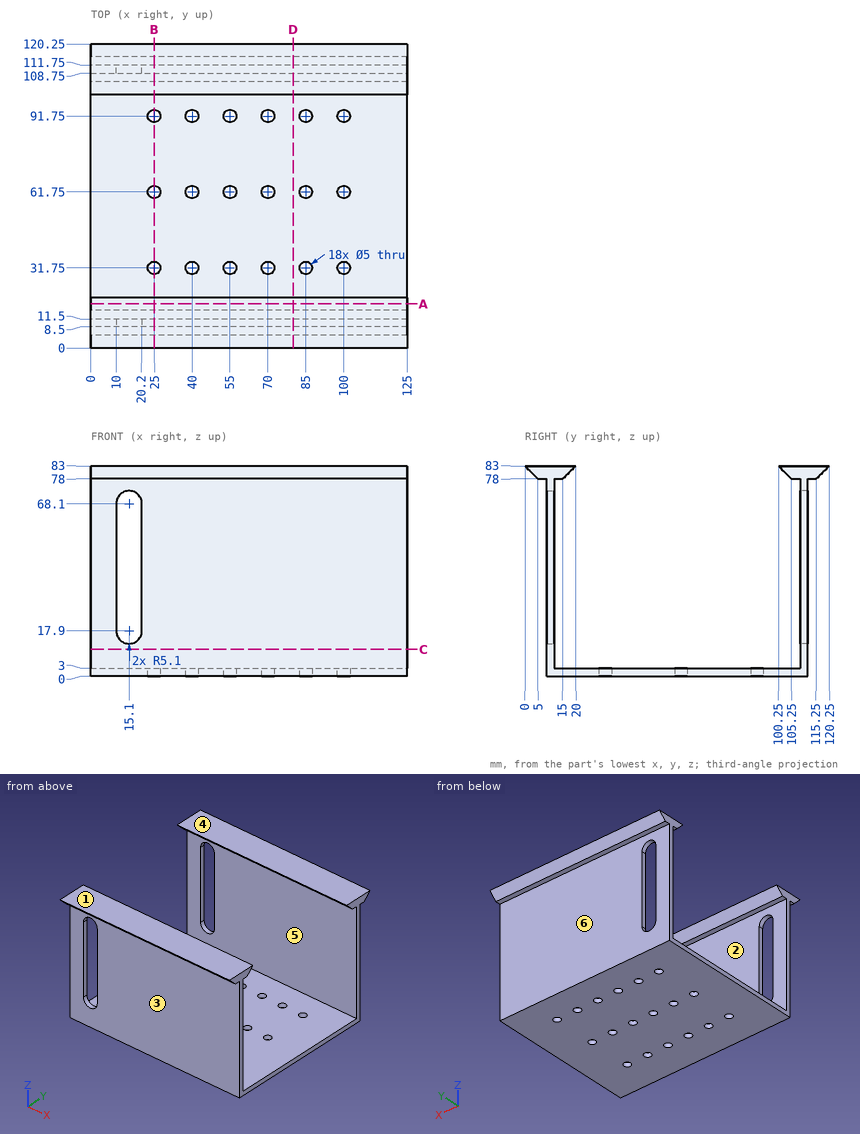
Source: three-view drawing plus pictorial views. Frame: mm from the lowest corner of the part. A direction names the side the tool comes from. Give positions to 0.01 mm unless a question says otherwise; leave off trailing zeros. Loops run counter-clockwise (first coordinate to the right, second up) from the corner with the lowest first, then second, coordinate; pieces in that order, holes last.
1) Reachability of the marked faces 4, 5 and 6 from +Z, -Z, +X, -X, +Y, -Y: full face, straight path, thin tool, end or side. Return the list, or none.
A:
face 4: +Z, +X, -X, +Y, -Y
face 5: +X, -X
face 6: -Z, +X, -X, +Y
2) Mould query, pull axis Y, two halves, no side actions, for the marked faces 1, 2 and 3. Classes: released by +Y, released by -Y, zero draft, split by the parting line, or undercut.
A:
face 1: zero draft
face 2: undercut
face 3: released by -Y
3) Line query: L1, parallel to Y at x = 25, z = 1.5; L2, parallel to Y at x = 42, z = 29.5; L3, parallel to Z at x = 67, y = 8. Output: solid intervals per line, ascending.
A:
L1: y = 8.5 to 29.25, 34.25 to 59.25, 64.25 to 89.25, 94.25 to 111.75
L2: y = 8.5 to 11.5, 108.75 to 111.75
L3: z = 78 to 83
4) Section query A-A on y = 17.5. Return the cut outline in (x, z), and give its area (4 significant figures).
A:
outline: (0, 0) - (125, 0) - (125, 3) - (0, 3) - close; (0, 80.5) - (125, 80.5) - (125, 83) - (0, 83) - close
area: 687.5 mm2
5) Section query D-D on x = 80. Return the cut outline in (y, z).
A:
outline: (0, 83) - (5, 78) - (8.5, 78) - (8.5, 0) - (111.75, 0) - (111.75, 78) - (115.25, 78) - (120.25, 83) - (100.25, 83) - (105.25, 78) - (108.75, 78) - (108.75, 3) - (11.5, 3) - (11.5, 78) - (15, 78) - (20, 83) - close
6) Section query C-C on z = 10.5. Return the cut outline in (x, y), and give its area (3 significant figures).
A:
outline: (0, 8.5) - (125, 8.5) - (125, 11.5) - (0, 11.5) - close; (0, 108.75) - (125, 108.75) - (125, 111.75) - (0, 111.75) - close
area: 750 mm2
7) Contact query for flat-ended pins moving along their axis: pin 1 (5 mm diameter, centred on x = 88, z = 58.5, fed in from +Y); pin 2 (6.5 mm diameter, centred on x = 85, y = 31.75, fed in from +Z); pin 3 (1 mm diameter, centred on x = 64.5, y = 114, fed in from -Z). Output: stop coordinate, or through.
A:
pin 1: stops at y = 111.75
pin 2: stops at z = 3
pin 3: stops at z = 78
8) Section query B-B on x = 25. Return the cut outline in (y, z), and give its area (3 significant figures).
A:
outline: (0, 83) - (5, 78) - (8.5, 78) - (8.5, 0) - (29.25, 0) - (29.25, 3) - (11.5, 3) - (11.5, 78) - (15, 78) - (20, 83) - close; (34.25, 0) - (59.25, 0) - (59.25, 3) - (34.25, 3) - close; (64.25, 0) - (89.25, 0) - (89.25, 3) - (64.25, 3) - close; (94.25, 0) - (111.75, 0) - (111.75, 78) - (115.25, 78) - (120.25, 83) - (100.25, 83) - (105.25, 78) - (108.75, 78) - (108.75, 3) - (94.25, 3) - close
area: 865 mm2
